from build123d import *

# Parameters (mm, degrees)
BOSS_EXTRUDE1_DEPTH = 3.175
SKETCH2_W           = 12.7
SKETCH2_H           = 6.35
CUT_EXTRUDE1_DEPTH  = 198.182581951
SKETCH3_W           = 19.05
SKETCH3_H           = 3.175
BOSS_EXTRUDE2_DEPTH = 6.35
SKETCH5_R           = 1.25
SKETCH5_R_2         = 0.6731
CUT_EXTRUDE3_DEPTH  = 198.182581951
SKETCH6_W           = 3.175
SKETCH6_H           = 44.45
CUT_EXTRUDE4_DEPTH  = 198.182581951


with BuildPart() as part:
    # Sketch1 → Boss-Extrude1 (new body)
    with BuildSketch(Plane(origin=(0, 0, 0), x_dir=(1, 0, 0), z_dir=(0, 1, 0))):
        Polygon((12.7, 0), (0, 0), (0, -50.8), (12.7, -50.8), (12.7, -47.625), (25.4, -47.625), (25.4, -50.8), (38.1, -50.8), (38.1, -47.625), (50.8, -47.625), (50.8, -50.8), (63.5, -50.8), (63.5, -47.625), (76.2, -47.625), (76.2, -50.8), (88.9, -50.8), (88.9, -47.625), (101.6, -47.625), (101.6, -50.8), (114.3, -50.8), (114.3, -47.625), (127, -47.625), (127, -50.8), (139.7, -50.8), (139.7, -47.625), (152.4, -47.625), (152.4, -50.8), (165.1, -50.8), (165.1, -47.625), (177.8, -47.625), (177.8, -50.8), (190.5, -50.8), (190.5, 0), (177.8, 0), (177.8, -3.175), (165.1, -3.175), (165.1, 0), (152.4, 0), (152.4, -3.175), (139.7, -3.175), (139.7, 0), (127, 0), (127, -3.175), (114.3, -3.175), (114.3, 0), (101.6, 0), (101.6, -3.175), (88.9, -3.175), (88.9, 0), (76.2, 0), (76.2, -3.175), (63.5, -3.175), (63.5, 0), (50.8, 0), (50.8, -3.175), (38.1, -3.175), (38.1, 0), (25.4, 0), (25.4, -3.175), (12.7, -3.175), align=None)
    extrude(amount=BOSS_EXTRUDE1_DEPTH)

    # Sketch2 → Cut-Extrude1 (cut, through all)
    with BuildSketch(Plane(origin=(0, 3.175, 0), x_dir=(1, 0, 0), z_dir=(0, 1, 0))):
        with Locations((6.35, -25.4)):
            Rectangle(SKETCH2_W, SKETCH2_H)
    extrude(amount=-CUT_EXTRUDE1_DEPTH, mode=Mode.SUBTRACT)

    # Sketch3 → Boss-Extrude2 (add)
    with BuildSketch(Plane.ZY):
        with Locations((12.7, 1.5875)):
            Rectangle(SKETCH3_W, SKETCH3_H)
        with Locations((38.1, 1.5875)):
            Rectangle(SKETCH3_W, SKETCH3_H)
    extrude(amount=BOSS_EXTRUDE2_DEPTH)

    # Sketch5 → Cut-Extrude3 (cut, through all)
    with BuildSketch(Plane(origin=(0, 3.175, 0), x_dir=(1, 0, 0), z_dir=(0, 1, 0))):
        with Locations(Location((131.425, -17.9, 0), (0, 0, 270))):
            Circle(SKETCH5_R)
        with Locations(Location((131.425, -32.9, 0), (0, 0, 270))):
            Circle(SKETCH5_R)
        with Locations(Location((112.375, -21.0566, 0), (0, 0, 270))):
            Circle(SKETCH5_R_2)
        with Locations(Location((112.375, -29.7434, 0), (0, 0, 270))):
            Circle(SKETCH5_R_2)
        with Locations(Location((93.325, -29.7434, 0), (0, 0, 270))):
            Circle(SKETCH5_R_2)
        with Locations(Location((93.325, -21.0566, 0), (0, 0, 270))):
            Circle(SKETCH5_R_2)
        with Locations(Location((161.925, -32.9, 0), (0, 0, 270))):
            Circle(SKETCH5_R)
        with Locations(Location((161.925, -17.9, 0), (0, 0, 270))):
            Circle(SKETCH5_R)
    extrude(amount=-CUT_EXTRUDE3_DEPTH, mode=Mode.SUBTRACT)

    # Sketch6 → Cut-Extrude4 (cut, through all)
    with BuildSketch(Plane(origin=(0, 3.175, 0), x_dir=(1, 0, 0), z_dir=(0, 1, 0))):
        with Locations((-4.7625, -25.4)):
            Rectangle(SKETCH6_W, SKETCH6_H)
    extrude(amount=-CUT_EXTRUDE4_DEPTH, mode=Mode.SUBTRACT)


solid = part.part
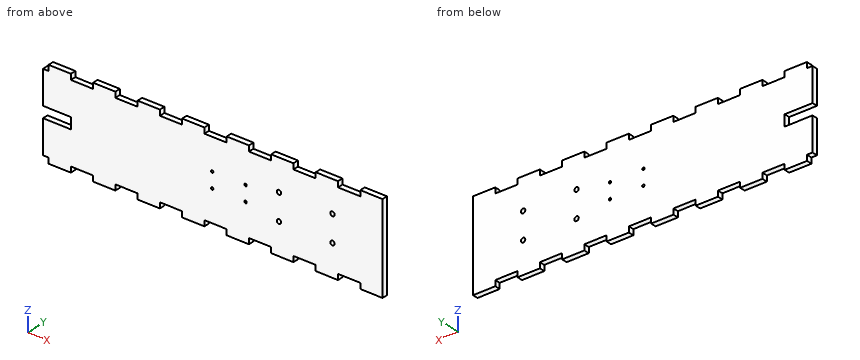
Input: part model. Units: mm. Frame: model coordinates. Give positions to 0.01 mm unless a question says otherwise; leave off trailing zeros. Order: outer loops, then holes, each group sorted by start corner. A loop starts at its lowest first (then second) coordinate and runs counter-clockwise, first axis right, second up.
Q1. Ray query, probe 1 along X at (y, z) = (0.75, 17.9) (3 decimals); probe 2 along Z at (x, y) = (12.5, 0.4) (3 decimals); probe 3 along Z at (x, y) = (148, 2.65) (3 decimals). Return the intervals inside material, ascending.
Checked values:
probe 1: x = -3.175 to 130.175, 132.675 to 160.675, 163.175 to 190.5
probe 2: z = 0 to 22.225, 28.575 to 50.8
probe 3: z = 3.175 to 47.625
Q2. Section B-B on y = 2.15. State how many separate pieces and enclosed holes the cut face has, and give its area (3 significant figures).
Checked values:
separate pieces: 1
enclosed holes: 8
area: 9,130 mm2
Q3. Section A-A on x = 124. Output: boundary loops of the cut face in (y, z) (3 decimals), and give its area (3 significant figures).
Checked values:
outline: (0, 3.175) - (3.175, 3.175) - (3.175, 47.625) - (0, 47.625) - close
area: 141 mm2
Q4. Contact query for flat-ended pins moving along their axis: pin 1 Ø1.6 at (x, y) = (17, 1) entering from -Z (3 decimals); pin 2 Ø1 at (x, y) = (22, 1) entering from +Z (3 decimals); pin 3 Ø1.8 at (x, z) = (112.38, 21.06) entering from -Y; pin 4 Ø1.6 at (y, z) = (1.5, 49) entering from -X. Output: stop coordinate, or through.
Checked values:
pin 1: stops at z = 3.175
pin 2: stops at z = 47.625
pin 3: stops at y = 0
pin 4: stops at x = 0
